Input: part model. Units: mm. Frame: model coordinates. A direction names the side the tool comes from. Round coordinates to 2 decimals unless told otherwise and drop trailing zeros. Write each loop counter-clockwise with the first axis right and the second up, starting at its lowest first coordinate (ties: lowest second). Pieces come first, ordered by that corner, then holes. Notation, with made-up numbers: (-2, 82) -> (25, 82) arc R18 cw to (25, 113) -> close; hole circle Ø2 at (54.5, -37.5). An arc over 180 degrees is marked (long way). Use CSV: the item, a comma, the result in double quotes.
```python
from build123d import *

# Parameters (mm, degrees)
F0_W     = 80
F0_H     = 47.3202
F0_R     = 12.2174
F1_DEPTH = 51.0794
F2_DEPTH = 12.7
F3_R     = 5.08
F4_R     = 5.08


with BuildPart() as f1:
    # F0 (on Front) → F1 (new body)
    with BuildSketch(Plane.XZ):
        with Locations((-11.767063, 24.444504)):
            Rectangle(F0_W, F0_H)
        with Locations((-11.929573, 23.557259)):
            Circle(F0_R, mode=Mode.SUBTRACT)
    extrude(amount=F1_DEPTH)

    # F0 (on Front) → F2 (join)
    with BuildSketch(Plane.XZ):
        with BuildLine():
            Line((28.232937, 0.784404), (-51.767063, 0.784404))
            ThreePointArc((-51.767063, 0.784404), (-11.767063, -39.215596), (28.232937, 0.784404))
        make_face()
    extrude(amount=F2_DEPTH)

    # F3
    f3_edges = [f1.edges().sort_by_distance(p)[0] for p in [
        (28.232937, -25.5397, 48.104604),
        (-11.767063, -51.0794, 0.784404),
        (-11.767063, -51.0794, 48.104604),
    ]]
    fillet(f3_edges, radius=F3_R)

    # F4
    f4_edges = [f1.edges().sort_by_distance(p)[0] for p in [
        (-14.307063, 0, 48.104604),
    ]]
    fillet(f4_edges, radius=F4_R)


solid = f1.part
```
Item 1: Section query D-D on y = -23. Return the cut outline in (x, z).
Worked answers:
outline,"(-51.77, 0.78) -> (28.23, 0.78) -> (28.23, 43.02) arc R5.08 ccw to (23.15, 48.1) -> (-51.77, 48.1) -> close; hole circle Ø24.43 at (-11.93, 23.56)"
Item 2: Pull-direction query (Z, two-part tool) for faces 3 (the face through (-12, -29, 0.784)), 4 (the face through (-11.21, -49.55, 46.66)), 5 (the face through (-50.24, -1.45, 24.78)), 6 (the face through (-14.58, -25.18, 11.63)); classes: +Z half, -Z half, draft (parallel to the pull), parting line (faces both ways), or undercut.
Worked answers:
face 3,"-Z half"
face 4,"+Z half"
face 5,"draft"
face 6,"undercut"
Item 3: Section query B-B on y = -7. Return the cut outline in (x, z), plus the area to 3 significant figures.
Worked answers:
outline,"(-51.77, 0.78) arc R40 ccw to (28.23, 0.78) -> (28.23, 43.02) arc R5.08 ccw to (23.15, 48.1) -> (-51.77, 48.1) -> close; hole circle Ø24.43 at (-11.93, 23.56)"
area,"5,820 mm²"
Item 4: Section query A-A on z = 17. Return the cut outline in (x, y), plus the area to 3 significant figures.
Worked answers:
outline,"(-51.77, -51.08) -> (-22.24, -51.08) -> (-22.24, 0) -> (-46.69, 0) arc R5.08 ccw to (-51.77, -5.08) -> close; (-1.62, -51.08) -> (28.23, -51.08) -> (28.23, -5.08) arc R5.08 ccw to (23.15, 0) -> (-1.62, 0) -> close"
area,"3,020 mm²"
Item 5: Set-up query: faces 1 (the face through (28.233, -28, 22)), 2 (the face through (-12, -12.7, -14)). Return all of +Z, -Z, +X, -X, +Y, -Y with unobstructed straight access to the full face (end or side cutting, diameter ignored); none if empty.
Worked answers:
face 1,"+Z, -Z, +X, +Y, -Y"
face 2,"-Z, +X, -X, -Y"
Item 6: First-contact query: pin 1 Ø8 at (x, y) = (12.5, -42.5) entering from -Z; pin 2 Ø1.5 at (y, z) = (-9.5, -25) entering from -X. Flat tips, straight axial feed; report the tip coordinate or a pass-through.
Worked answers:
pin 1,"stops at z = 0.78"
pin 2,"stops at x = -42.96"
Item 7: Line query: line 1 (Z direction, x = -12.5, y = -9.5); line 2 (X direction, y = -36, z = 15); line 3 (Z direction, x = -1, y = -44). Output: solid intervals per line, ascending.
Worked answers:
line 1,"z = -39.21 to 11.35, 35.76 to 48.1"
line 2,"x = -51.77 to -20.65, -3.21 to 28.23"
line 3,"z = 0.78 to 18.1, 29.02 to 48.1"
Item 8: Section query C-C on z = 28. Return the cut outline in (x, y), plus the area to 3 significant figures.
Worked answers:
outline,"(-51.77, -51.08) -> (-23.31, -51.08) -> (-23.31, 0) -> (-46.69, 0) arc R5.08 ccw to (-51.77, -5.08) -> close; (-0.55, -51.08) -> (28.23, -51.08) -> (28.23, -5.08) arc R5.08 ccw to (23.15, 0) -> (-0.55, 0) -> close"
area,"2,910 mm²"
